Could you check a few things on this model? Use its own coordinates, in mm. A direction names the side the tool comes from. Coordinates: 2 decimals unless noted, no trailing zeros. Write each loop counter-clockwise with the first axis right and the second up, starting at its lowest first coordinate (ties: lowest second). Pieces come first, ordered by that corner, then holes.
```python
from build123d import *

# Parameters (mm, degrees)
F0_R     = 4
F0_R_2   = 1.5
F1_DEPTH = 2
F3_DEPTH = 2
F4_R     = 2.5
F4_R_2   = 1.5
F5_DEPTH = 2.5
F6_R     = 0.4


with BuildPart() as f1:
    # F0 (on Front) → F1 (new body)
    with BuildSketch(Plane.XZ):
        Circle(F0_R)
        Circle(F0_R_2, mode=Mode.SUBTRACT)
    extrude(amount=F1_DEPTH)

    # F2 (on face) → F3 (join, through all)
    with BuildSketch(Plane.XZ.offset(2)):
        Polygon((0.439486, 5.412983), (0, 5.412983), (-0.439486, 5.412983), (-1, 3.872983), (1, 3.872983), align=None)
        Polygon((-3.087098, 4.468038), (-2.802517, 2.854102), (-1.070466, 3.854102), (-2.325886, 4.907524), (-2.706492, 4.687781), align=None)
        Polygon((-4.907524, 2.325886), (-3.854102, 1.070466), (-2.854102, 2.802517), (-4.468038, 3.087098), (-4.687781, 2.706492), align=None)
        Polygon((-5.412983, -0.439486), (-3.872983, -1), (-3.872983, 1), (-5.412983, 0.439486), (-5.412983, 0), align=None)
        Polygon((-4.468038, -3.087098), (-2.854102, -2.802517), (-3.854102, -1.070466), (-4.907524, -2.325886), (-4.687781, -2.706492), align=None)
        Polygon((-2.325886, -4.907524), (-1.070466, -3.854102), (-2.802517, -2.854102), (-3.087098, -4.468038), (-2.706492, -4.687781), align=None)
        Polygon((0.439486, -5.412983), (1, -3.872983), (-1, -3.872983), (-0.439486, -5.412983), (0, -5.412983), align=None)
        Polygon((3.087098, -4.468038), (2.802517, -2.854102), (1.070466, -3.854102), (2.325886, -4.907524), (2.706492, -4.687781), align=None)
        Polygon((4.907524, -2.325886), (3.854102, -1.070466), (2.854102, -2.802517), (4.468038, -3.087098), (4.687781, -2.706492), align=None)
        Polygon((5.412983, 0.439486), (3.872983, 1), (3.872983, -1), (5.412983, -0.439486), (5.412983, 0), align=None)
        Polygon((4.468038, 3.087098), (2.854102, 2.802517), (3.854102, 1.070466), (4.907524, 2.325886), (4.687781, 2.706492), align=None)
        Polygon((2.325886, 4.907524), (1.070466, 3.854102), (2.802517, 2.854102), (3.087098, 4.468038), (2.706492, 4.687781), align=None)
    extrude(amount=-F3_DEPTH)

    # F4 (on face) → F5 (join)
    with BuildSketch(Plane(origin=(0, 0, 0), x_dir=(-1, 0, 0), z_dir=(0, 1, 0))):
        Circle(F4_R)
        Circle(F4_R_2, mode=Mode.SUBTRACT)
    extrude(amount=F5_DEPTH)

    # F6
    f6_edges = [f1.edges().sort_by_distance(p)[0] for p in [
        (2.325886, -1, 4.907524),
        (3.087098, -1, 4.468038),
        (4.468038, -1, 3.087098),
        (4.907524, -1, 2.325886),
        (5.412983, -1, 0.439486),
        (5.412983, -1, -0.439486),
        (4.907524, -1, -2.325886),
        (4.468038, -1, -3.087098),
        (3.087098, -1, -4.468038),
        (2.325886, -1, -4.907524),
        (0.439486, -1, -5.412983),
        (-0.439486, -1, -5.412983),
        (-2.325886, -1, -4.907524),
        (-3.087098, -1, -4.468038),
        (-4.468038, -1, -3.087098),
        (-4.907524, -1, -2.325886),
        (-5.412983, -1, -0.439486),
        (-5.412983, -1, 0.439486),
        (-4.907524, -1, 2.325886),
        (-4.468038, -1, 3.087098),
        (-3.087098, -1, 4.468038),
        (-2.325886, -1, 4.907524),
        (-0.439486, -1, 5.412983),
        (0.439486, -1, 5.412983),
    ]]
    fillet(f6_edges, radius=F6_R)


solid = f1.part
```
Item 1: If we mould it in two halves opening along Z, with no side actions, what happens to faces 5 (the flat face through (-4.52, -1.014, -0.764)), 6 (the flat face through (-1.28, 0, -2.33)), 7 (the flat face through (0.77, -1.01, 4.5))? For each: released by +Z, released by -Z, zero draft, split by the parting line, or undercut.
Item 2: If I drill on line 1 along Z through (x, y) = (4.25, -0.7); line 2 along Z through (x, y) = (0, 1.25); line 3 along Z through (x, y) = (0, -1.05), over which ranges is the centre line in solid material (lowest first)?
Item 3: I want a section at C-C, the plane y = 2.2. List the corners of the cut face in (x, z) for me.
Item 4: Will these pins go through, and if not, where does the flat tip stop? pin 1 Ø1.5 at (x, y) = (-1, 1) entering from +Z; pin 2 Ø2.5 at (x, z) = (0, 0) entering from -Y; pin 3 Ø1 at (x, y) = (-2, -0.5) entering from -Z.
Item 5: I want a section at A-A, the plane z = 0. List the corners of the cut face in (x, y) for me.
Item 6: Which directions (+Z, -Z, +X, -X, +Y, -Y) give clear straight access to the entire face, cutting with the end or side of a thin tool? Please do faces 1 (the flat face through (-4.3, -1, -1.6)), 2 (the flat face through (4.3, -1, 1.6)), 3 (the flat face through (1.6, -1, -4.3)), 4 (the flat face through (1.6, -1, 4.3)).
Item 7: I want a section at B-B, the plane x = 0. List the corners of the cut face in (y, z) for me.
Item 8: I want a section at D-D, the plane x = -2.25. List the corners of the cut face in (y, z) for me, then the cut area to 3 significant figures.
Taken from the geometry:
1. face 5: undercut
1. face 6: zero draft
1. face 7: released by +Z
2. line 1: z = -3.04 to -1.54, -0.86 to 0.86, 1.54 to 3.04
2. line 2: z = -2.5 to -1.5, 1.5 to 2.5
2. line 3: z = -5.41 to -1.5, 1.5 to 5.41
3. outline: circle Ø5 at (0, 0); hole circle Ø3 at (0, 0)
4. pin 1: stops at z = 2.49
4. pin 2: passes through
4. pin 3: stops at z = -4.82
5. outline: (-5.41, -2) - (-1.5, -2) - (-1.5, 2.5) - (-2.5, 2.5) - (-2.5, 0) - (-5.41, 0) - close; (1.5, -2) - (5.41, -2) - (5.41, 0) - (2.5, 0) - (2.5, 2.5) - (1.5, 2.5) - close
6. face 1: -X, +Y, -Y
6. face 2: +X, +Y, -Y
6. face 3: -Z, +Y, -Y
6. face 4: +Z, +Y, -Y
7. outline: (-2, -5.41) - (0, -5.41) - (0, -2.5) - (2.5, -2.5) - (2.5, -1.5) - (-2, -1.5) - close; (-2, 1.5) - (2.5, 1.5) - (2.5, 2.5) - (0, 2.5) - (0, 5.41) - (-2, 5.41) - close
8. outline: (-2, -4.8) - (0, -4.8) - (0, -1.09) - (2.5, -1.09) - (2.5, 1.09) - (0, 1.09) - (0, 4.8) - (-2, 4.8) - close
8. area: 24.7 mm2
